```python
from build123d import *

# Parameters (mm, degrees)
F0_W      = 99.1851314902
F0_H      = 82.2389237583
F1_DEPTH  = 58.8
F2_W      = 37.8797464073
F2_H      = 22.678008303
F3_DEPTH  = 53
F4_W      = 14.9525329471
F4_H      = 10.2175623178
F5_DEPTH  = 23.2
F6_W      = 15.9493666142
F6_H      = 10.7159819454
F6_W_2    = 16.6969913989
F6_H_2    = 10.9651889652
F6_W_3    = 14.9525329471
F6_H_3    = 12.4604459852
F7_DEPTH  = 25
F8_W      = 37.8797464073
F8_H      = 22.678008303
F9_DEPTH  = 3
F10_W     = 5.9913191944
F10_H     = 4.6931989491
F10_W_2   = 1.7973957583
F10_H_2   = 1.597687602
F10_W_3   = 6.5904529765
F10_W_4   = 1.497827936
F10_H_3   = 1.0984092951
F10_W_5   = 5.6917527691
F10_H_4   = 2.2966712713
F10_H_5   = 4.4934898615
F10_W_6   = 21.2691789493
F10_H_6   = 2.1968167275
F10_W_7   = 6.690306589
F10_H_7   = 1.5976838768
F10_H_8   = 1.6975402832
F11_DEPTH = 6
F12_W     = 12.4604427256
F12_H     = 7.2270575911
F13_DEPTH = 25


with BuildPart() as f1:
    # F0 (on Top) → F1 (new body)
    with BuildSketch(Plane.XY):
        with Locations((0.4984177649, 2.741297707)):
            Rectangle(F0_W, F0_H)
    extrude(amount=F1_DEPTH)

    # F2 (on face) → F3 (join)
    with BuildSketch(Plane.YZ.offset(50.09098351)):
        with Locations((2.4920888245, 29.2820418254)):
            Rectangle(F2_W, F2_H)
    extrude(amount=F3_DEPTH)

    # F4 (on face) → F5 (join)
    with BuildSketch(Plane(origin=(0, 0, 0), x_dir=(1, 0, 0), z_dir=(0, 0, -1))):
        with Locations((-34.0518206358, 25.7931184024)):
            Rectangle(F4_W, F4_H)
    extrude(amount=F5_DEPTH)

    # F6 (on face) → F7 (join)
    with BuildSketch(Plane(origin=(0, 0, 0), x_dir=(1, 0, 0), z_dir=(0, 0, -1))):
        with Locations((34.2314103618, 26.0423282161)):
            Rectangle(F6_W, F6_H)
        with Locations((33.8575979695, -31.64952714)):
            Rectangle(F6_W_2, F6_H_2)
        with Locations((-34.0518206358, -31.64952714)):
            Rectangle(F6_W_3, F6_H_3)
    extrude(amount=F7_DEPTH)

    # F8 (on face) → F9 (join)
    with BuildSketch(Plane.YZ.offset(103.09098351)):
        with Locations((2.4920888245, 29.2820418254)):
            Rectangle(F8_W, F8_H)
    extrude(amount=F9_DEPTH)

    # F10 (on face) → F11 (join)
    with BuildSketch(Plane.YZ.offset(106.09098351)):
        with Locations((-11.5880584344, 34.5423240215)):
            Rectangle(F10_W, F10_H)
        with Locations((-11.6879125126, 34.4923958182)):
            Rectangle(F10_W_2, F10_H_2, mode=Mode.SUBTRACT)
        with Locations((16.3714285009, 34.5423240215)):
            Rectangle(F10_W_3, F10_H)
        with Locations((17.1203424688, 34.3426130712)):
            Rectangle(F10_W_4, F10_H_3, mode=Mode.SUBTRACT)
        with Locations((-11.0388533212, 25.7550571114)):
            Rectangle(F10_W_5, F10_H_4)
        with Locations((-11.0388533212, 22.359976545)):
            Rectangle(F10_W_5, F10_H_5)
        with Locations((2.441612538, 22.359976545)):
            Rectangle(F10_W_6, F10_H_5)
        with Locations((16.3714285009, 25.7051298395)):
            Rectangle(F10_W_3, F10_H_6)
        with Locations((16.3714285009, 22.359976545)):
            Rectangle(F10_W_3, F10_H_5)
        with Locations((-11.5381302312, 39.0857402235)):
            Rectangle(F10_W_7, F10_H_7)
        with Locations((16.3714285009, 38.8361029327)):
            Rectangle(F10_W_3, F10_H_8)
    extrude(amount=F11_DEPTH)

    # F12 (on face) → F13 (join)
    with BuildSketch(Plane(origin=(-49.0941479802, 0, 0), x_dir=(0, -1, 0), z_dir=(-1, 0, 0))):
        with Locations((-0.7476268802, 11.8374209851)):
            Rectangle(F12_W, F12_H)
    extrude(amount=F13_DEPTH)


solid = f1.part
```
For this review, take the finished solid that the model builds, in its own axes (mm). A direction names the side the tool comes from. Round coordinates to 2 decimals unless told otherwise and drop trailing zeros. Loops run counter-clockwise (first coordinate to the right, second up) from the corner with the lowest first, then second, coordinate; pieces in that order, holes last.
Q1. Machinability: for faces 1 (the face through (78, -16.448, 29)), 2 (the face through (78, 2, 40.621)), 3 (the face through (-61, 1, 8.224)), which of the approach directions +Z, -Z, +X, -X, +Y, -Y give a long, thin tool a straight path to every point of the face, cutting with its end or side? Answer none if there is none.
Result sheet:
face 1: +Z, -Z, +X, -Y
face 2: +Z, +X, +Y, -Y
face 3: -Z, -X, +Y, -Y
Q2. Mouldability with a two-part tool opening along Y and no side actions: class faces 4 (the face through (-26.576, -26, -11)), 5 (the face through (34, 26.167, -12)), 6 (the face through (109, -13.885, 24)), 7 (the face through (-34, 25.419, -12)) as +Y half, -Y half, draft (parallel to the pull), parting line (faces both ways), or undercut.
Result sheet:
face 4: draft
face 5: undercut
face 6: -Y half
face 7: undercut
Q3. Insertion check: pin 1 Ø1 at (y, z) = (17.5, 12) entering from +X; pin 2 Ø0.5 at (x, y) = (110, -11.5) entering from +Z; pin 3 Ø1.2 at (x, z) = (109, 34.5) entering from +Y. Each pin has a flat end and moves straight along its axis. Give the tip position at first contact, or say it passes through.
Result sheet:
pin 1: stops at x = 50.09
pin 2: stops at z = 39.88
pin 3: stops at y = 19.67
Q4. Add section B-B on x = 34.5. Write out the cut boundary in (y, z).
Result sheet:
outline: (-38.38, 0) - (-31.4, 0) - (-31.4, -25) - (-20.68, -25) - (-20.68, 0) - (26.17, 0) - (26.17, -25) - (37.13, -25) - (37.13, 0) - (43.86, 0) - (43.86, 58.8) - (-38.38, 58.8) - close
Q5. Add section A-A on z = -18. Write out the cut boundary in (x, y), plus the area to 3 significant figures.
Result sheet:
outline: (-41.53, -30.9) - (-26.58, -30.9) - (-26.58, -20.68) - (-41.53, -20.68) - close; (-41.53, 25.42) - (-26.58, 25.42) - (-26.58, 37.88) - (-41.53, 37.88) - close; (25.51, 26.17) - (42.21, 26.17) - (42.21, 37.13) - (25.51, 37.13) - close; (26.26, -31.4) - (42.21, -31.4) - (42.21, -20.68) - (26.26, -20.68) - close
area: 693 mm2
Q6. To check wall thickness, follow line 1 along X through (y, z) = (-28.5, -1); line 2 along X through (y, z) = (37, 33.5); line 3 along Z through (x, y) = (96.5, -11). State the ranges of each line that lie inside material, in increasing order.
Result sheet:
line 1: x = -41.53 to -26.58, 26.26 to 42.21
line 2: x = -49.09 to 50.09
line 3: z = 17.94 to 40.62
Q7. Add section D-D on z = 3.5. Write out the cut boundary in (x, y), plus the area to 3 significant figures.
Result sheet:
outline: (-49.09, -38.38) - (50.09, -38.38) - (50.09, 43.86) - (-49.09, 43.86) - close
area: 8,160 mm2
Q8. Add section C-C on y = 28. Write out the cut boundary in (x, z), plus the area to 3 significant figures.
Result sheet:
outline: (-49.09, 0) - (-41.53, 0) - (-41.53, -25) - (-26.58, -25) - (-26.58, 0) - (25.51, 0) - (25.51, -25) - (42.21, -25) - (42.21, 0) - (50.09, 0) - (50.09, 58.8) - (-49.09, 58.8) - close
area: 6,620 mm2
